Verification items for this drawing (mm, ordinates from the low corner). A direction names the side the tool comes from. Round coordinates to 2 decimals unless told otherwise and drop trailing zeros. Loops run counter-clockwise (first coordinate to the right, second up) from the corner with the lowest first, then second, coordinate; pieces in that order, holes last. Notation, with made-up numbers: (44, 68) - (82, 68) arc R29 cw to (82, 90) - close; hole circle Ø3 at (36.5, 12.5). An arc over 180 degrees is marked (long way). Write item = value, one per line.
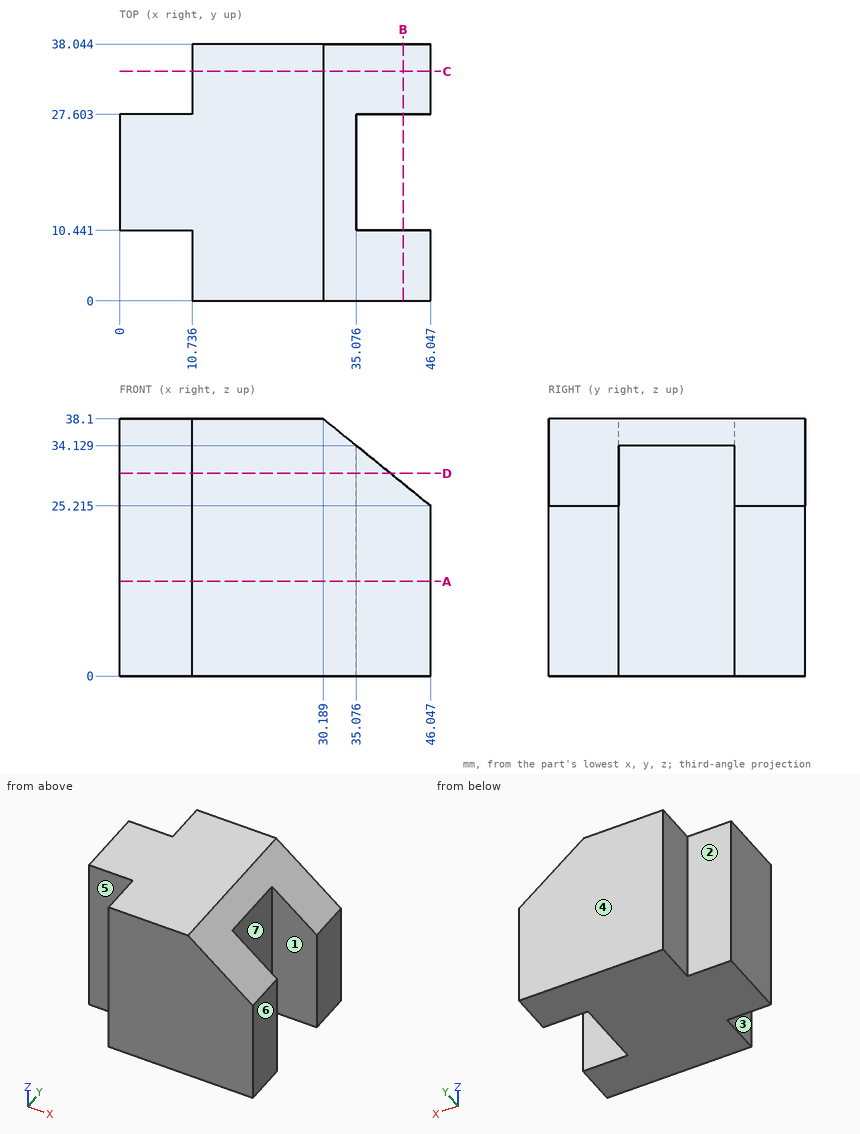
(1) Section check B-B (x = 42). Enter the section's corners in (y, z) (1 decimal), then the cut area to 3 significant figures.
Answers follow:
outline = (0, 0) - (10.4, 0) - (10.4, 28.5) - (0, 28.5) - close; (27.6, 0) - (38, 0) - (38, 28.5) - (27.6, 28.5) - close
area = 595 mm²
(2) Scan lines: L1, parallel to Y at x = 36, z = 18.5 (1 decimal); L2, parallel to X at y = 20.5, z = 3 (1 decimal); L3, parallel to X at y = 34, z = 19.5 (1 decimal). Record each from-to range of solid material in increasing order. Write a range as [from, to].
Answers follow:
L1 = [0, 10.4], [27.6, 38]
L2 = [0, 35.1]
L3 = [10.7, 46]
(3) Set-up check for the marked faces 1, 2, 3 and 4: record each of +Z, -Z, +X, -X, +Y, -Y from which the full face is reachable in a straight line by a thin tool's end or side.
Answers follow:
face_1 = +Z, -Z, +X
face_2 = +Z, -Z, -X, +Y
face_3 = +Z, -Z, -X, -Y
face_4 = +Z, -Z, +X, -X, +Y
(4) Mould release check, pull along Y, two halves, no side actions. Record for the marked faces 5, 6 and 7: pulls with the +Y half, pulls with the -Y half, needs draft (parallel to the pull), parting line crosses it, or undercut.
Answers follow:
face_5 = pulls with the -Y half
face_6 = needs draft
face_7 = undercut
(5) Section check D-D (z = 30). Enter the section's corners in (x, y) (1 decimal), then the cut area to 3 significant figures.
Answers follow:
outline = (0, 10.4) - (10.7, 10.4) - (10.7, 0) - (40.2, 0) - (40.2, 10.4) - (35.1, 10.4) - (35.1, 27.6) - (40.2, 27.6) - (40.2, 38) - (10.7, 38) - (10.7, 27.6) - (0, 27.6) - close
area = 1,220 mm²
(6) Section check C-C (y = 34). Enter the section's corners in (x, z) (1 decimal), then the cut area to 3 significant figures.
Answers follow:
outline = (10.7, 0) - (46, 0) - (46, 25.2) - (30.2, 38.1) - (10.7, 38.1) - close
area = 1,240 mm²
(7) Section check A-A (z = 14). Enter the section's corners in (x, y) (1 decimal).
Answers follow:
outline = (0, 10.4) - (10.7, 10.4) - (10.7, 0) - (46, 0) - (46, 10.4) - (35.1, 10.4) - (35.1, 27.6) - (46, 27.6) - (46, 38) - (10.7, 38) - (10.7, 27.6) - (0, 27.6) - close
(8) Gauge pin test, flat ends, axial feed: pin 1 (3 mm diameter, centred on y = 31.5, z = 23.5, fed in from -X); pin 2 (8 mm diameter, centred on y = 18, z = 7.5, fed in from +X); pin 3 (3 mm diameter, centred on x = 4.5, z = 27, fed in from -Y). Record the tip position at first contact, or that the pin passes through.
Answers follow:
pin_1 = 10.74
pin_2 = 35.08
pin_3 = 10.44
